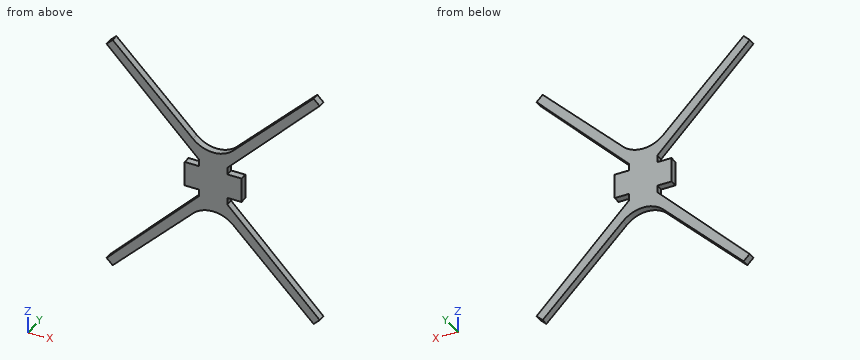
from build123d import *

# Parameters (mm, degrees)
SKETCH1_W           = 25.4
SKETCH1_H           = 11.176
BOSS_EXTRUDE1_DEPTH = 3.175


with BuildPart() as part:
    # Sketch1 → Boss-Extrude1 (new body)
    with BuildSketch(Plane(origin=(0, 0, 0), x_dir=(1, 0, 0), z_dir=(0, 1, 0))):
        with Locations((12.7, 5.588)):
            Rectangle(SKETCH1_W, SKETCH1_H)
        with BuildLine():
            Line((19.05, 11.176), (19.05, 14.351))
            Line((19.05, 14.351), (60.326216075, 56.589419985))
            Line((60.326216075, 56.589419985), (57.601280605, 59.252280605))
            Line((57.601280605, 59.252280605), (21.680256121, 23.331256121))
            ThreePointArc((21.680256121, 23.331256121), (12.7, 19.611512242), (3.719743879, 23.331256121))
            Line((3.719743879, 23.331256121), (-32.201280605, 59.252280605))
            Line((-32.201280605, 59.252280605), (-34.926216075, 56.589419985))
            Line((-34.926216075, 56.589419985), (6.35, 14.351))
            Line((6.35, 14.351), (6.35, 11.176))
            Line((6.35, 11.176), (19.05, 11.176))
        make_face()
        with BuildLine():
            Line((19.05, 0), (19.05, -3.175))
            Line((19.05, -3.175), (60.326216075, -45.413419985))
            Line((60.326216075, -45.413419985), (57.601280605, -48.076280605))
            Line((57.601280605, -48.076280605), (21.680256121, -12.155256121))
            ThreePointArc((21.680256121, -12.155256121), (12.7, -8.435512242), (3.719743879, -12.155256121))
            Line((3.719743879, -12.155256121), (-32.201280605, -48.076280605))
            Line((-32.201280605, -48.076280605), (-34.926216075, -45.413419985))
            Line((-34.926216075, -45.413419985), (6.35, -3.175))
            Line((6.35, -3.175), (6.35, 0))
            Line((6.35, 0), (19.05, 0))
        make_face()
    extrude(amount=BOSS_EXTRUDE1_DEPTH)


solid = part.part
Could you check a few things on this model? Use its own coordinates, in mm. Coordinates: 2 decimals unless noted, no trailing zeros. Loops run counter-clockwise (first coordinate to the right, second up) from the corner with the lowest first, then second, coordinate; pieces in that order, holes last.
1. Imagine slicing it at A-A (z = 41.5). Please give me the cut outline in (x, y) (3 decimals).
2. For P1, Ø1, axis at x = -25.5, y = 2, coming from the -Z side; P2, Ø1.6, axis at y = 2, z = 2, coming from the +X side; P3, Ø1.6, axis at y = 1.5, z = -4, coming from the +X side, each with a flat end and sliding along its axis, tell me the tip position at first contact or that it passes through.
3. Imagine slicing it at C-C (y = 0.9). Please give me the cut outline in (x, z) (3 decimals), and give its area (3 significant figures).
4. Imagine slicing it at B-B (x = -8). Please give me the cut outline in (y, z) (3 decimals), and give its area (3 significant figures).
5. Imagine slicing it at D-D (z = -2). Please give me the cut outline in (x, y) (3 decimals).
6. I need wall thicknesses on L1, parallel to Z at x = 22.5, y = 0.9 (3 decimals); L2, parallel to X at y = 2.15, z = 34.5 (3 decimals); L3, parallel to X at y = 1.4, z = -50. Which ranges of each line are inside material? Lowest first, please.
Computed values:
1. outline: (-31.102, 0) - (-25.625, 0) - (-25.625, 3.175) - (-31.102, 3.175) - close; (51.025, 0) - (56.502, 0) - (56.502, 3.175) - (51.025, 3.175) - close
2. P1: stops at z = -53.05
2. P2: stops at x = 19.05
2. P3: stops at x = 25.4
3. outline: (-34.926, -56.589) - (-32.201, -59.252) - (3.72, -23.331) arc R12.7 cw to (21.68, -23.331) - (57.601, -59.252) - (60.326, -56.589) - (19.05, -14.351) - (19.05, -11.176) - (25.4, -11.176) - (25.4, 0) - (19.05, 0) - (19.05, 3.175) - (60.326, 45.413) - (57.601, 48.076) - (21.68, 12.155) arc R12.7 cw to (3.72, 12.155) - (-32.201, 48.076) - (-34.926, 45.413) - (6.35, 3.175) - (6.35, 0) - (0, 0) - (0, -11.176) - (6.35, -11.176) - (6.35, -14.351) - close
3. area: 1,450 mm2
4. outline: (0, -35.051) - (3.175, -35.051) - (3.175, -29.036) - (0, -29.036) - close; (0, 17.86) - (3.175, 17.86) - (3.175, 23.875) - (0, 23.875) - close
4. area: 38.2 mm2
5. outline: (0, 0) - (25.4, 0) - (25.4, 3.175) - (0, 3.175) - close
6. L1: z = -24.151 to -17.881, -11.176 to 0, 6.705 to 12.975
6. L2: x = -24.261 to -18.625, 44.025 to 49.661
6. L3: x = -28.49 to -22.95, 48.35 to 53.89
